from build123d import *

# Parameters (mm, degrees)
SKETCH1_W           = 80
SKETCH1_H           = 20
BOSS_EXTRUDE1_DEPTH = 10
SKETCH2_R           = 2.5
CUT_EXTRUDE1_DEPTH  = 47.813641243
SKETCH3_W           = 25
SKETCH3_H           = 1
CUT_EXTRUDE2_DEPTH  = 47.813641243


with BuildPart() as part:
    # Sketch1 → Boss-Extrude1 (new body)
    with BuildSketch(Plane.XY):
        with Locations((-0.372188153, 11.484958231)):
            Rectangle(SKETCH1_W, SKETCH1_H)
    extrude(amount=BOSS_EXTRUDE1_DEPTH)

    # Sketch2 → Cut-Extrude1 (cut, through all)
    with BuildSketch(Plane.XY.offset(10)):
        with Locations((-23.942188153, 12.584958231)):
            Circle(SKETCH2_R)
        with Locations(Location((23.197811847, 12.584958231, 0), (0, 0, 180))):
            Circle(SKETCH2_R)
    extrude(amount=-CUT_EXTRUDE1_DEPTH, mode=Mode.SUBTRACT)

    # Sketch3 → Cut-Extrude2 (cut, through all)
    with BuildSketch(Plane.XY.offset(10)):
        with Locations((-0.372188153, 18.984958231)):
            Rectangle(SKETCH3_W, SKETCH3_H)
    extrude(amount=-CUT_EXTRUDE2_DEPTH, mode=Mode.SUBTRACT)


solid = part.part
The model under review builds one solid part; all positions refer to its coordinate system, in mm. A direction names the side the tool comes from. Coordinates: 2 decimals unless noted, no trailing zeros. Write each loop counter-clockwise with the first axis right and the second up, starting at its lowest first coordinate (ties: lowest second). Pieces come first, ordered by that corner, then holes. Notation, with made-up numbers: (42, 51.25) - (75, 51.25) arc R5 cw to (75, 56.25) - close; hole circle Ø3 at (56.25, 44). An arc over 180 degrees is marked (long way). Answer as CSV lines item,"result".
(1) Clearance check with a flat-ended pin moving along its axis: pin 1 Ø4 at (x, y) = (-5, 15) entering from -Z. State where the tip first meets the part, or that it passes through.
Data:
pin 1,"stops at z = 0"
(2) We need section B-B (y = 11.5). Give the boundary of the cut face in (x, z), plus the area to 3 significant figures.
Data:
outline,"(-40.37, 0) - (-26.19, 0) - (-26.19, 10) - (-40.37, 10) - close; (-21.69, 0) - (20.95, 0) - (20.95, 10) - (-21.69, 10) - close; (25.45, 0) - (39.63, 0) - (39.63, 10) - (25.45, 10) - close"
area,"710 mm2"
(3) Tool access review of faces 1 (the flat face through (-1, 12, 0)), 2 (the flat face through (-1, 19.485, 5)): name each direction out of +Z, -Z, +X, -X, +Y, -Y from which nothing blocks a thin tool from reaching the whole face with its end or side.
Data:
face 1,"-Z, +X, -X, +Y, -Y"
face 2,"+Z, -Z"
(4) For line 1 along X through (y, z) = (12.75, 5.25); line 2 along X through (y, z) = (10.5, 3.75); line 3 along Y through (x, z) = (8.5, 1.25), list the stretches that pass through material, from the lowest coordinate up. Write a range as [from, to].
Data:
line 1,"x = [-40.37, -26.44], [-21.45, 20.7], [25.69, 39.63]"
line 2,"x = [-40.37, -25.32], [-22.56, 21.82], [24.58, 39.63]"
line 3,"y = [1.48, 18.48], [19.48, 21.48]"
(5) We need section C-C (z = 3.75). Give the boundary of the cut face in (x, y), plus the area to 3 significant figures.
Data:
outline,"(-40.37, 1.48) - (39.63, 1.48) - (39.63, 21.48) - (-40.37, 21.48) - close; hole circle Ø5 at (-23.94, 12.58); hole (-12.87, 18.48) - (12.13, 18.48) - (12.13, 19.48) - (-12.87, 19.48) - close; hole circle Ø5 at (23.2, 12.58)"
area,"1,540 mm2"
(6) We need section A-A (x = -3.5). Give the boundary of the cut face in (y, z), plus the area to 3 significant figures.
Data:
outline,"(1.48, 0) - (18.48, 0) - (18.48, 10) - (1.48, 10) - close; (19.48, 0) - (21.48, 0) - (21.48, 10) - (19.48, 10) - close"
area,"190 mm2"
(7) Mouldability with a two-part tool opening along X and no side actions: class faces 3 (the cylindrical face through (-22.598, 14.693, 5.07)), 4 (the flat face through (39.628, 11, 5)), 5 (the flat face through (-1, 1.485, 5)), 6 (the flat face through (-40.372, 11, 5)) as pulls with the +X half, pulls with the -X half, needs draft (parallel to the pull), parting line crosses it, or undercut.
Data:
face 3,"undercut"
face 4,"pulls with the +X half"
face 5,"needs draft"
face 6,"pulls with the -X half"
